```python
from build123d import *

# Parameters (mm, degrees)
SKETCH1_W               = 25.4
SKETCH1_H               = 25.4
BOSS_EXTRUDE1_DEPTH     = 79.375
SKETCH2_W               = 19.05
SKETCH2_H               = 53.975
CUT_EXTRUDE1_DEPTH      = 20.6375
CUT_EXTRUDE2_DEPTH      = 88.124684361
CUT_EXTRUDE2_DEPTH_BACK = 88.124684361
SKETCH3_R               = 2.38125
CUT_EXTRUDE3_DEPTH      = 88.124684361
CUT_EXTRUDE3_DEPTH_BACK = 88.124684361
SKETCH4_R               = 2.38125
CUT_EXTRUDE4_DEPTH      = 59.055
CUT_EXTRUDE4_DEPTH_BACK = 5.08
SKETCH6_R               = 3.81
SKETCH8_R               = 2.38125
CUT_EXTRUDE5_DEPTH      = 6.35


with BuildPart() as part:
    # Sketch1 → Boss-Extrude1 (new body)
    with BuildSketch(Plane.XY):
        with Locations((12.7, 12.7)):
            Rectangle(SKETCH1_W, SKETCH1_H)
    extrude(amount=BOSS_EXTRUDE1_DEPTH)

    # Sketch2 → Cut-Extrude1 (cut)
    with BuildSketch(Plane(origin=(0, 25.4, 0), x_dir=(1, 0, 0), z_dir=(0, 1, 0))):
        with Locations((15.875, -39.6875)):
            Rectangle(SKETCH2_W, SKETCH2_H)
    extrude(amount=-CUT_EXTRUDE1_DEPTH, mode=Mode.SUBTRACT)

    # Sketch3 → Cut-Extrude2 (cut, two sides: drawn at the far end of the back side and taken through both)
    with BuildSketch(Plane.ZY.offset(-CUT_EXTRUDE2_DEPTH_BACK)):
        with Locations((26.9875, 12.7)):
            Circle(SKETCH3_R)
        with Locations((39.6875, 12.7)):
            Circle(SKETCH3_R)
        with Locations((52.3875, 12.7)):
            Circle(SKETCH3_R)
    extrude(amount=CUT_EXTRUDE2_DEPTH + CUT_EXTRUDE2_DEPTH_BACK, mode=Mode.SUBTRACT)

    # Sketch4 → Cut-Extrude3 (cut, two sides: drawn at the far end of the back side and taken through both)
    with BuildSketch(Plane.XZ.offset(-CUT_EXTRUDE3_DEPTH_BACK)):
        with Locations(Location((12.7, 52.3875, 0), (0, 0, 270))):
            Circle(SKETCH4_R)
        with Locations(Location((12.7, 39.6875, 0), (0, 0, 270))):
            Circle(SKETCH4_R)
        with Locations(Location((12.7, 26.9875, 0), (0, 0, 270))):
            Circle(SKETCH4_R)
    extrude(amount=CUT_EXTRUDE3_DEPTH + CUT_EXTRUDE3_DEPTH_BACK, mode=Mode.SUBTRACT)

    # Sketch6 → Cut-Extrude4 (cut, two sides: drawn at the far end of the back side and taken through both)
    with BuildSketch(Plane.XY.offset(12.7).offset(-CUT_EXTRUDE4_DEPTH_BACK)):
        with Locations((22.225, 15.08125)):
            Circle(SKETCH6_R)
    extrude(amount=CUT_EXTRUDE4_DEPTH + CUT_EXTRUDE4_DEPTH_BACK, mode=Mode.SUBTRACT)

    # Sketch8 → Cut-Extrude5 (cut)
    with BuildSketch(Plane(origin=(25.4, 0, 0), x_dir=(0, 0, -1), z_dir=(1, 0, 0))):
        with Locations((-73.025, 15.08125)):
            Circle(SKETCH8_R)
        with Locations((-6.35, 15.08125)):
            Circle(SKETCH8_R)
    extrude(amount=-CUT_EXTRUDE5_DEPTH, mode=Mode.SUBTRACT)


solid = part.part
```
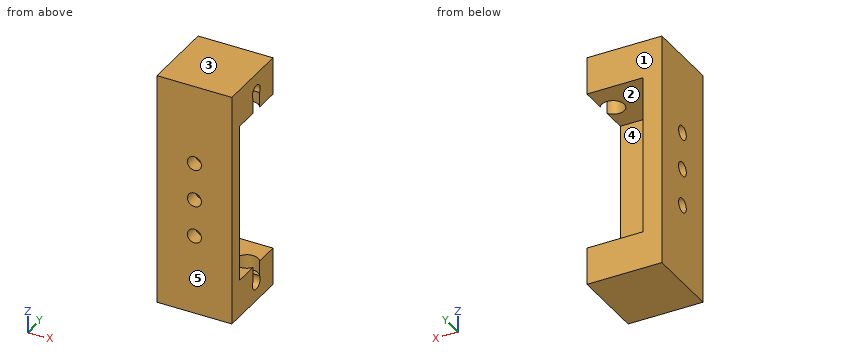
Part model, mm, in its own coordinate system. Face numbers are marked on the shaded views. A direction names the side the tool comes from. Round coordinates to 2 decimals unless told otherwise and drop trailing zeros. Write each loop counter-clockwise with the first axis right and the second up, starting at its lowest first coordinate (ties: lowest second). Pieces come first, ordered by that corner, then holes. Notation, with made-up numbers: M 87.25,-12.5 L 114.25,-12.5 A24 ccw 114.25,1.5 Z; hole C 61.25,26 d7. An arc over 180 degrees is marked long. Answer as CSV lines item,"result". Start each with the question number.
1) Band-saw the part on A-A (x = 12.7). List the corners of the cut face in (y, z) (1 decimal), then the cut area to 3 significant figures.
2) Which spindle directions (+Z, -Z, +X, -X, +Y, -Y) get a long thin tool onto all of the face, cutting with end or side? Do the marked faces 4 and 5. Say none if no direction does.
3) Band-saw the part on B-B (y = 3.25). List the corners of the cut face in (x, z) (1 decimal).
4) Band-saw the part on C-C (y = 9.5). List the corners of the cut face in (x, z) (3 decimals).
5) Drill centre lines: L1, parallel to Z at x = 23, y = 20.25 (3 decimals); L2, parallel to X at y = 14.5, z = 45; L3, parallel to Y at x = 13, z = 32. Where is each one in solid material? Low to high.
6) Drop flat-ended pins along their axis: pin 1 (5.5 mm diameter, centred on y = 12.7, z = 52.39, fed in from +X); pin 2 (5.5 mm diameter, centred on x = 13, z = 37.5, fed in from +Y); pin 3 (4.5 mm diameter, centred on x = 12.7, z = 52.39, fed in from -Y). Give the stop position or say it passes through.
7) Mould opens along Z. For the marked faces 1, 2 and 3 say: +Z half, -Z half, draft (parallel to the pull), parting line (faces both ways), or undercut.
Worked out:
1,outline,"M 0,0 L 25.4,0 L 25.4,12.7 L 4.8,12.7 L 4.8,24.6 L 0,24.6 Z; M 0,29.4 L 4.8,29.4 L 4.8,37.3 L 0,37.3 Z; M 0,42.1 L 4.8,42.1 L 4.8,50 L 0,50 Z; M 0,54.8 L 4.8,54.8 L 4.8,66.7 L 25.4,66.7 L 25.4,79.4 L 0,79.4 Z"
1,area,"834 mm²"
2,face 4,"+X, +Y"
2,face 5,"+Z, -Z, +X, -X, -Y"
3,outline,"M 0,0 L 25.4,0 L 25.4,79.4 L 0,79.4 Z; hole C 12.7,27 d4.8; hole C 12.7,39.7 d4.8; hole C 12.7,52.4 d4.8"
4,outline,"M 0,0 L 25.4,0 L 25.4,12.7 L 6.35,12.7 L 6.35,66.675 L 25.4,66.675 L 25.4,79.375 L 0,79.375 Z"
5,L1,"0 to 12.7, 66.675 to 79.375"
5,L2,"0 to 6.35"
5,L3,"0 to 4.76"
6,pin 1,"x = 6.35"
6,pin 2,"y = 4.76"
6,pin 3,"through"
7,face 1,"draft"
7,face 2,"undercut"
7,face 3,"+Z half"
